Model file for the job. Use its own axes, mm. Round coordinates to 2 decimals unless told otherwise and drop trailing zeros. Answer as CSV lines item,"result".
```python
from build123d import *

# Parameters (mm, degrees)
SKETCH003_R  = 120
PAD001_DEPTH = 35
SKETCH002_R  = 150.91951
PAD_DEPTH    = 35


with BuildPart() as pad001:
    # Sketch003 → Pad001 (new body, symmetric)
    with BuildSketch(Plane.XZ):
        with Locations((-1.007223, -112)):
            Circle(SKETCH003_R)
    extrude(amount=PAD001_DEPTH, both=True)


with BuildPart() as pad:
    # Sketch002 → Pad (new body, symmetric)
    with BuildSketch(Plane.XZ):
        with Locations((-1.007223, -146)):
            Circle(SKETCH002_R)
    extrude(amount=PAD_DEPTH, both=True)


with BuildPart() as common:
    # Sketch001 → Loft section 0
    with BuildSketch(Plane.XY.offset(8)):
        with BuildLine():
            Line((-31.000014, 16.191998), (-31.000014, -21.808002))
            ThreePointArc((-31.000014, -21.808002), (-29.974879, -24.282877), (-27.500001, -25.308002))
            Line((-27.500001, -25.308002), (27.499999, -25.308002))
            ThreePointArc((27.499999, -25.308002), (29.974879, -24.282877), (31.000014, -21.808002))
            Line((31.000014, -21.808002), (31.000014, 16.191998))
            ThreePointArc((31.000014, 16.191998), (29.974879, 18.666873), (27.499999, 19.691998))
            Line((27.499999, 19.691998), (-27.500001, 19.691998))
            ThreePointArc((-27.500001, 19.691998), (-29.974879, 18.666873), (-31.000014, 16.191998))
        make_face()
    # Sketch → Loft section 1
    with BuildSketch(Plane.XY):
        with BuildLine():
            Line((-38.586045, 14.832981), (-38.586045, -22.167019))
            ThreePointArc((-38.586045, -22.167019), (-35.339018, -30.006036), (-27.5, -33.253064))
            Line((-27.5, -33.253064), (27.5, -33.253064))
            ThreePointArc((27.5, -33.253064), (35.339018, -30.006036), (38.586045, -22.167019))
            Line((38.586045, -22.167019), (38.586045, 14.832981))
            ThreePointArc((38.586045, 14.832981), (35.339018, 22.671999), (27.5, 25.919026))
            Line((27.5, 25.919026), (-27.5, 25.919026))
            ThreePointArc((-27.5, 25.919026), (-35.339018, 22.671999), (-38.586045, 14.832981))
        make_face()
    loft()

    # Cut: cut Pad
    add(pad.part, mode=Mode.SUBTRACT)

    # Common: intersect Pad001
    add(pad001.part, mode=Mode.INTERSECT)


solid = common.part
```
Q1. Flat gauge pins, fed straight in: pin 1 (1 mm diameter, centred on x = 20, y = -25, fed in from +Z); pin 2 (5 mm diameter, centred on x = -30, y = 6, fed in from +Z). Where does each tip first touch, or does it go through?
Checks:
pin 1,"z = 6.23"
pin 2,"z = 5.04"
Q2. Mould opens along X. For faces 1 (the cylindrical face through (-0.034, -3.85, 4.916)), 2 (the cylindrical face through (1.023, -3.575, 7.983)) say: +X half, -X half, draft (parallel to the pull), parting line (faces both ways), or undercut.
Checks:
face 1,"undercut"
face 2,"parting line"
Q3. Wall check: L1, parallel to Z at x = 35, y = 7; L2, parallel to Z at x = -33.5, y = -11.5; L3, parallel to Y at x = 15, z = 6.5. Give the ranges that are in metal, low to high. Write a range as [from, to].
Checks:
L1,"[0.56, 2.47]"
L2,"[1.38, 3.52]"
L3,"[-26.8, 20.86]"
